The drawing under review shows one solid part. Ordinate dimensions are in mm from its lowest x, y, z. A direction names the side the tool comes from. Round coordinates to 2 decimals unless told otherwise and drop trailing zeros. Loops run counter-clockwise (first coordinate to the right, second up) from the corner with the lowest first, then second, coordinate; pieces in that order, holes last. Notation, with made-up numbers: (79.5, 82) - (125.5, 82) arc R12 ccw to (125.5, 96) - close; hole circle Ø3 at (33.25, -27). An arc over 180 degrees is marked (long way). Answer as CSV lines item,"result".
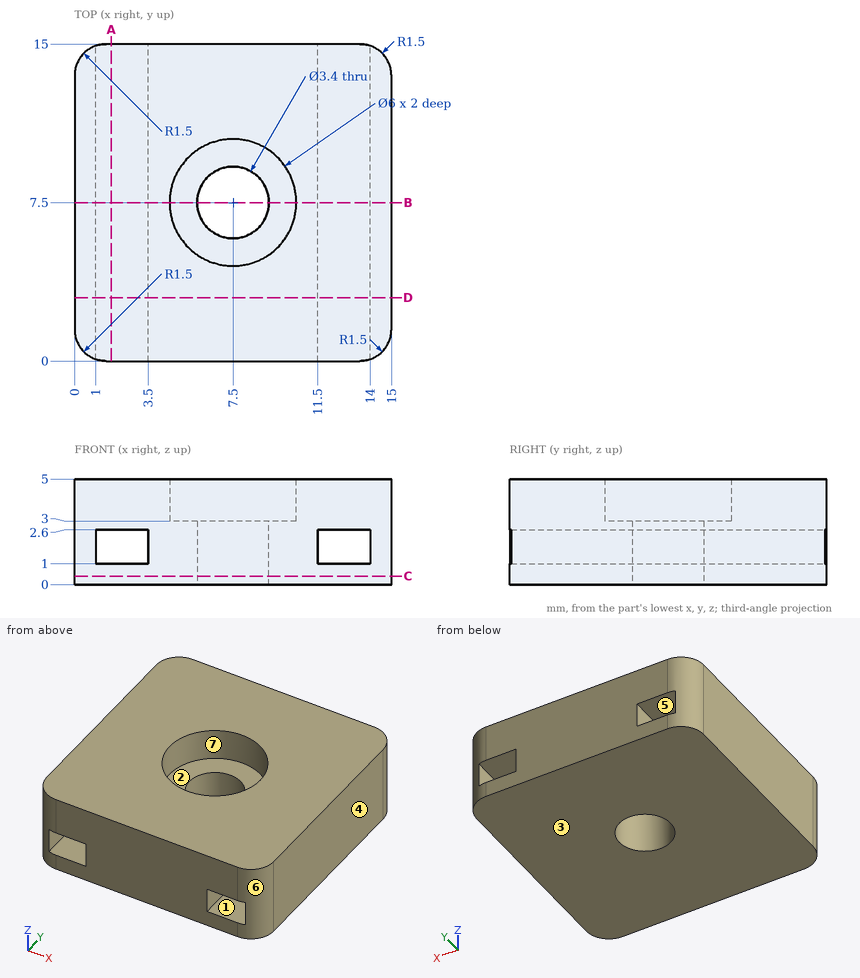
1. Wall thickness on probe 1 along X at (y, z) = (7.5, 1.5); probe 2 along Y at (x, z) = (7.5, 4.4); probe 3 along X at (y, z) = (14.5, 2.15): over which ranges is each line inside the solid? List them lowest first.
Numbers:
probe 1,"x = 0 to 1, 3.5 to 5.8, 9.2 to 11.5, 14 to 15"
probe 2,"y = 0 to 4.5, 10.5 to 15"
probe 3,"x = 0.38 to 1, 3.5 to 11.5, 14 to 14.62"
2. Take a section at B-B (y = 7.5). State the section outline as (x, z) points.
Numbers:
outline,"(0, 0) - (5.8, 0) - (5.8, 3) - (4.5, 3) - (4.5, 5) - (0, 5) - close; (9.2, 0) - (15, 0) - (15, 5) - (10.5, 5) - (10.5, 3) - (9.2, 3) - close; hole (1, 1) - (3.5, 1) - (3.5, 2.6) - (1, 2.6) - close; hole (11.5, 1) - (14, 1) - (14, 2.6) - (11.5, 2.6) - close"
3. Draft analysis for pull direction Z (two halves, no side actions). For the marked faces 1, 2, 3 and 4, state which applies: +Z half, -Z half, draft (parallel to the pull), parting line (faces both ways), or undercut.
Numbers:
face 1,"undercut"
face 2,"+Z half"
face 3,"-Z half"
face 4,"draft"
4. Clearance check with a flat-ended pin moving along its axis: pin 1 (1.8 mm diameter, centred on x = 6.5, y = 6, fed in from +Z). State where the tip first meets the part, or that it passes through.
Numbers:
pin 1,"stops at z = 3"
5. Tool access review of the marked faces 5, 6 and 7: name each direction out of +Z, -Z, +X, -X, +Y, -Y from which nothing blocks a thin tool from reaching the whole face with its end or side.
Numbers:
face 5,"+Y, -Y"
face 6,"+Z, -Z, +X, -Y"
face 7,"+Z"
6. Take a section at D-D (y = 3). State the section outline as (x, z) points.
Numbers:
outline,"(0, 0) - (15, 0) - (15, 5) - (0, 5) - close; hole (1, 1) - (3.5, 1) - (3.5, 2.6) - (1, 2.6) - close; hole (11.5, 1) - (14, 1) - (14, 2.6) - (11.5, 2.6) - close"
7. Take a section at C-C (z = 0.4). State the section outline as (x, y) points.
Numbers:
outline,"(0, 1.5) arc R1.5 ccw to (1.5, 0) - (13.5, 0) arc R1.5 ccw to (15, 1.5) - (15, 13.5) arc R1.5 ccw to (13.5, 15) - (1.5, 15) arc R1.5 ccw to (0, 13.5) - close; hole circle Ø3.4 at (7.5, 7.5)"
8. Take a section at A-A (x = 1.75). State the section outline as (y, z) points, plus the area to 3 significant figures.
Numbers:
outline,"(0, 0) - (15, 0) - (15, 1) - (0, 1) - close; (0, 2.6) - (15, 2.6) - (15, 5) - (0, 5) - close"
area,"51.0 mm²"
